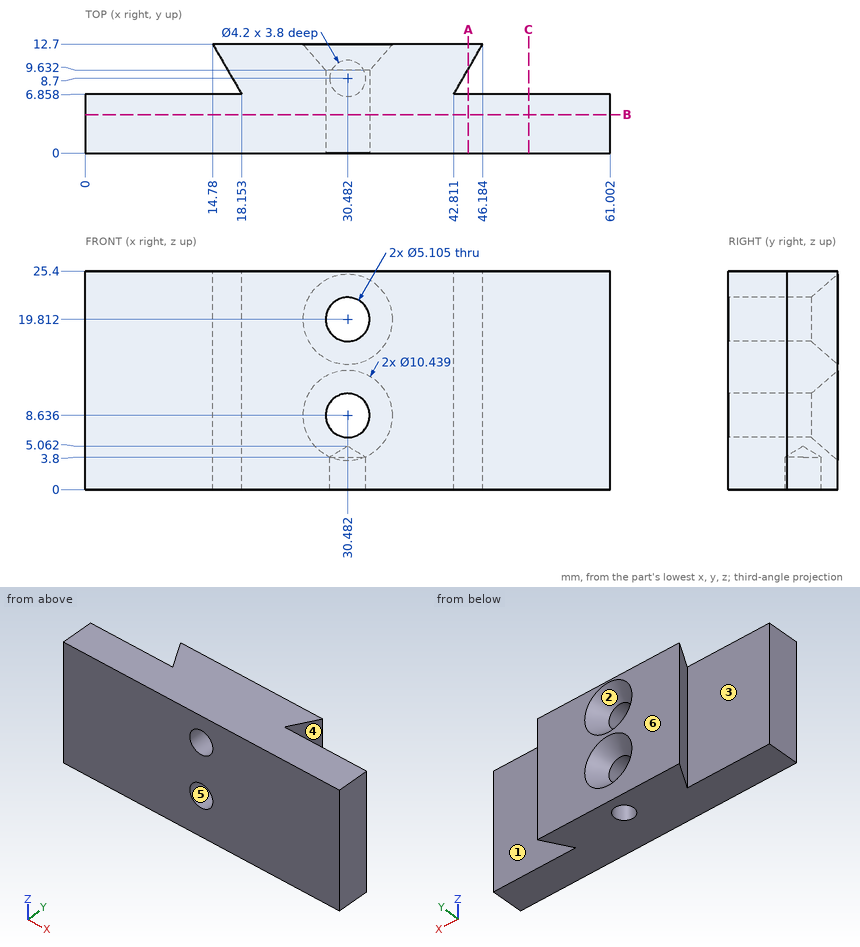
Part print with two shaded views. Sizes in mm from the minimum x, y, z corner. A direction names the side the tool comes from. Round coordinates to 2 decimals unless told otherwise and drop trailing zeros. Order: outer loops, then holes, each group sorted by start corner. A loop starts at its lowest first (then second) coordinate and runs counter-clockwise, first axis right, second up.
(1) Band-saw the part on A-A (x = 44.5). List the corners of the cut face in (y, z), then the cut area to 3 significant figures.
(2) Pull direction X, two halves, no side cores. Call the marked faces 4, 5 and 6: released by +X, released by -X, zero draft, split by the parting line, or undercut.
(3) Band-saw the part on C-C (x = 51.5). List the corners of the cut face in (y, z).
(4) Drill centre lines: line 1 (Z direction, x = 33, y = 11.75) (1 decimal); line 2 (Y direction, x = 7.5, z = 2.5); line 3 (X direction, y = 11.75, z = 22.25) (1 decimal). Where is each one in solid material? Low to high.
(5) Pin check, flat tips, straight feed: pin 1 (6.5 mm diameter, centred on x = 30.48, z = 8.64, fed in from +Y); pin 2 (1.5 mm diameter, centred on x = 10.5, z = 21, fed in from +Y). Stop position of each tip, or through.
(6) 3-axis set-ups, long thin cutter, end or side, ignore diameter. For the marked faces 1, 2 and 3: which of +Z, -Z, +X, -X, +Y, -Y reach the whole face in a straight line?
(7) Band-saw the part on B-B (y = 4.5). List the corners of the cut face in (x, z) (1 decimal), then the cut area to 3 significant figures.
Verdict:
1. outline: (0, 0) - (6.86, 0) - (6.86, 25.4) - (0, 25.4) - close; (9.78, 0) - (12.7, 0) - (12.7, 25.4) - (9.78, 25.4) - close
1. area: 248 mm2
2. face 4: released by +X
2. face 5: undercut
2. face 6: zero draft
3. outline: (0, 0) - (6.86, 0) - (6.86, 25.4) - (0, 25.4) - close
4. line 1: z = 0 to 5, 12.2 to 16.2, 23.4 to 25.4
4. line 2: y = 0 to 6.86
4. line 3: x = 15.3 to 26.8, 34.1 to 45.6
5. pin 1: stops at y = 10.44
5. pin 2: stops at y = 6.86
6. face 1: +Z, -Z, +X
6. face 2: +Y
6. face 3: +Z, -Z, -X
7. outline: (0, 0) - (61, 0) - (61, 25.4) - (0, 25.4) - close; hole circle Ø5.1 at (30.5, 8.6); hole circle Ø5.1 at (30.5, 19.8)
7. area: 1,510 mm2
